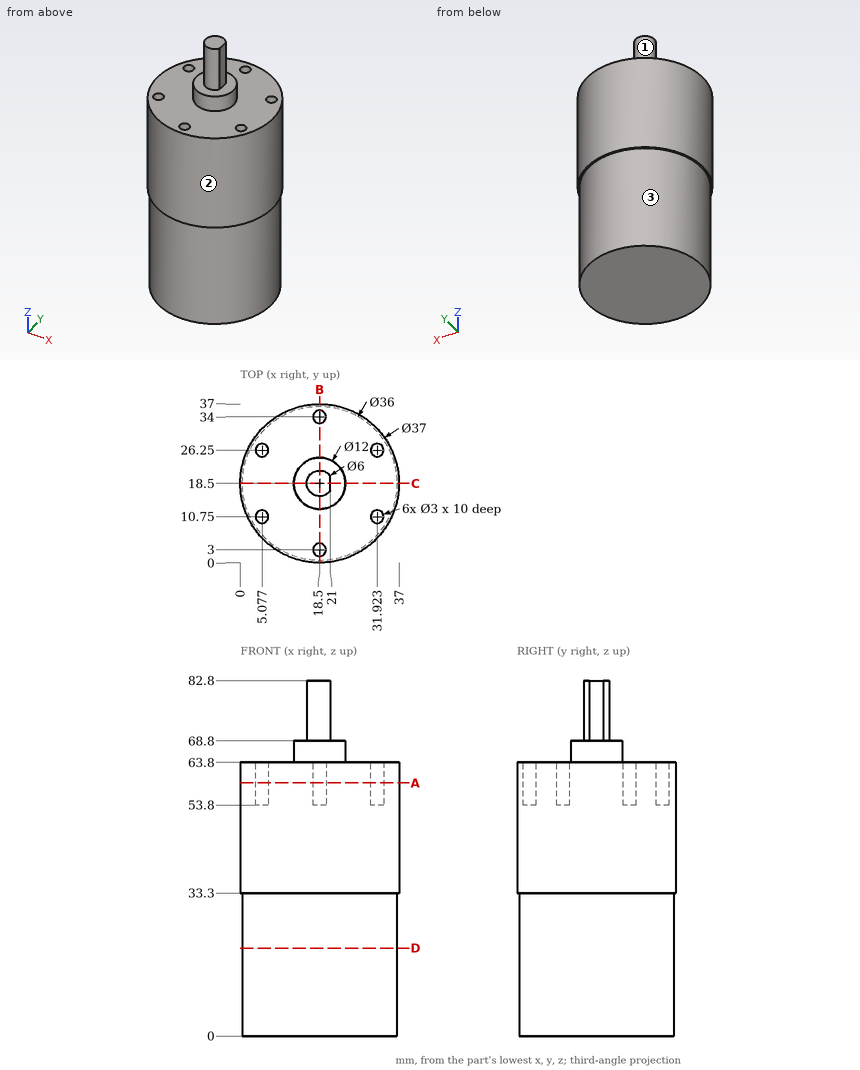
Answer from the drawing. Dimensions are ordinates in mm from the lowest x, y and z of the part. A direction names the side the tool comes from. Round coordinates to 2 decimals unless told otherwise and drop trailing zeros. Loops run counter-clockwise (first coordinate to the right, second up) from the corner with the lowest first, then second, coordinate; pieces in that order, holes last.
1) A cutting plane is placed at D-D on z = 20.5. Determine the outline of the cut face in (x, y), plus the area to 3 significant figures.
Outcome:
outline: circle Ø36 at (18.5, 18.5)
area: 1,020 mm2
2) A cutting plane is placed at B-B on x = 18.5. Determine the outline of the cut face in (y, z).
Outcome:
outline: (0, 33.3) - (0.5, 33.3) - (0.5, 0) - (36.5, 0) - (36.5, 33.3) - (37, 33.3) - (37, 63.8) - (35.5, 63.8) - (35.5, 53.8) - (32.5, 53.8) - (32.5, 63.8) - (24.5, 63.8) - (24.5, 68.8) - (21.5, 68.8) - (21.5, 82.8) - (15.5, 82.8) - (15.5, 68.8) - (12.5, 68.8) - (12.5, 63.8) - (4.5, 63.8) - (4.5, 53.8) - (1.5, 53.8) - (1.5, 63.8) - (0, 63.8) - close
3) A cutting plane is placed at C-C on y = 18.5. Determine the outline of the cut face in (x, z), plus the area to 3 significant figures.
Outcome:
outline: (0, 33.3) - (0.5, 33.3) - (0.5, 0) - (36.5, 0) - (36.5, 33.3) - (37, 33.3) - (37, 63.8) - (24.5, 63.8) - (24.5, 68.8) - (21, 68.8) - (21, 82.8) - (15.5, 82.8) - (15.5, 68.8) - (12.5, 68.8) - (12.5, 63.8) - (0, 63.8) - close
area: 2,460 mm2
4) Given P1, Ø1.5, axis at x = 18, y = 3, coming from the +Z side; P2, Ø12, axis at x = 19.5, z = 29.5, coming from the +Y side; P3, Ø10, axis at x = 25.5, z = 36.5, coming from the +Y side, each flat-ended and moving along its own axis, determine where each tip first touches the part or whether it passes through.
Outcome:
P1: stops at z = 53.8
P2: stops at y = 37
P3: stops at y = 36.89
5) A cutting plane is placed at A-A on z = 59. Determine the outline of the cut face in (x, y), plus the area to 3 significant figures.
Outcome:
outline: circle Ø37 at (18.5, 18.5); hole circle Ø3 at (5.08, 10.75); hole circle Ø3 at (5.08, 26.25); hole circle Ø3 at (18.5, 3); hole circle Ø3 at (18.5, 34); hole circle Ø3 at (31.92, 10.75); hole circle Ø3 at (31.92, 26.25)
area: 1,030 mm2
6) Consider line 1 (Y direction, x = 18.5, z = 60.75); line 2 (Y direction, x = 32.5, z = 59.5) (1 decimal); line 3 (X direction, y = 26, z = 61) (1 decimal). Determine where each line is inside the solid, lowest interval first.
Outcome:
line 1: y = 0 to 1.5, 4.5 to 32.5, 35.5 to 37
line 2: y = 6.4 to 9.4, 12.1 to 24.9, 27.6 to 30.6
line 3: x = 1.6 to 3.6, 6.6 to 30.4, 33.4 to 35.4
7) For the marked faces 1, 2 and 3, determine the directions among +Z, -Z, +X, -X, +Y, -Y from which every point of the face is accessible in a straight line to the end or side of a thin tool.
Outcome:
face 1: +Z
face 2: +Z, -Z
face 3: -Z
